Work out the finished part from the listing and answer in its coordinate system (mm). A direction names the side the tool comes from. Coordinates: 2 decimals unless noted, no trailing zeros. Order: outer loops, then holes, each group sorted by start corner. A loop starts at its lowest first (then second) coordinate and runs counter-clockwise, first axis right, second up. Notation, with made-up numbers: (-14.5, 79) -> (-2.5, 79) arc R19 cw to (-2.5, 90) -> close; hole circle Ø3 at (71.25, 16). An arc over 180 degrees is marked (long way). Write item = value, one per line. Start each with the question number.
Q1. The part is cut by section B-B, the plane z = -0.55. Determine the outline of the cut face in (x, y).
Q2. Straight lines are drawn through the part: L1, parallel to Y at x = 10.5, z = -0.85; L2, parallel to X at y = -12.75, z = -0.45; L3, parallel to Z at x = 11.25, y = 1. For each, find the intervals that lie inside material, in ascending order. Write a range as from..to.
Q3. Which of the six approach directions +Z, -Z, +X, -X, +Y, -Y give full straight-line access (tool end or side, diameter ignored) to faces 5 (the flat face through (9, -12, -0.9)), 6 (the flat face through (-0.1, 9.462, -0.5))?
Q4. The part is cut by section A-A, the plane y = 0.1. Determine the outline of the cut face in (x, z) (3 decimals).
Q5. The part is cut by section C-C, the plane y = -10.5. Determine the outline of the cut face in (x, z) (3 decimals).
Q6. Flat-ended cylindrical pins translate along their axes: pin 1 (2 mm diameter, centred on x = -10.5, y = -0.5, fed in from -Z); pin 2 (1.3 mm diameter, centred on x = -9.5, y = 0.5, fed in from +Z). Find the tip coordinate at first contact, or state that the pin passes through.
Q7. For a pull along Y with two mould halves and no side action, classify faces 1 (the flat face through (9, 0, -0.9)), 2 (the flat face through (0, -2, -0.975)), 3 (the flat face through (-9, -12, 0)), 4 (the cylindrical face through (11.9, -13.83, -0.46)) as +Y half, -Y half, draft (parallel to the pull), parting line (faces both ways), or undercut.
```python
from build123d import *

# Parameters (mm, degrees)
SKETCH3_W           = 25
SKETCH3_H           = 23.862
BOSS_EXTRUDE1_DEPTH = 0.9
FILLET1_R           = 2
SKETCH4_R           = 1.1
CUT_EXTRUDE1_DEPTH  = 20.089787846
BOSS_EXTRUDE2_DEPTH = 0.075
BOSS_EXTRUDE3_START = 0.075
BOSS_EXTRUDE3_DEPTH = 0.075


with BuildPart() as part:
    # Sketch3 → Boss-Extrude1 (new body)
    with BuildSketch(Plane.XY):
        with Locations((0, -2.469)):
            Rectangle(SKETCH3_W, SKETCH3_H)
    extrude(amount=-BOSS_EXTRUDE1_DEPTH)

    # Fillet1
    fillet1_edges = [part.edges().sort_by_distance(p)[0] for p in [
        (-12.5, 9.462, -0.45),
        (12.5, 9.462, -0.45),
        (12.5, -14.4, -0.45),
        (-12.5, -14.4, -0.45),
    ]]
    fillet(fillet1_edges, radius=FILLET1_R)

    # Sketch4 → Cut-Extrude1 (cut, through all)
    with BuildSketch(Plane.XY):
        with Locations((-10.5, 0.1)):
            Circle(SKETCH4_R)
        with Locations((-10.5, -12.4)):
            Circle(SKETCH4_R)
        with Locations((10.5, -12.4)):
            Circle(SKETCH4_R)
        with Locations((10.5, 0.1)):
            Circle(SKETCH4_R)
    extrude(amount=-CUT_EXTRUDE1_DEPTH, mode=Mode.SUBTRACT)

    # Sketch5 → Boss-Extrude2 (add)
    with BuildSketch(Plane.XY):
        with BuildLine():
            Line((12.5, 1.426649916), (12.5, 7.462))
            ThreePointArc((12.5, 7.462), (11.914213562, 8.876213562), (10.5, 9.462))
            Line((10.5, 9.462), (-10.5, 9.462))
            ThreePointArc((-10.5, 9.462), (-11.914213562, 8.876213562), (-12.5, 7.462))
            Line((-12.5, 7.462), (-12.5, 1.426649916))
            ThreePointArc((-12.5, 1.426649916), (-8.1, 0.1), (-12.5, -1.226649916))
            Line((-12.5, -1.226649916), (-12.5, -11.073350084))
            ThreePointArc((-12.5, -11.073350084), (-8.802943725, -10.702943725), (-9.173350084, -14.4))
            Line((-9.173350084, -14.4), (9.173350084, -14.4))
            ThreePointArc((9.173350084, -14.4), (8.802943725, -10.702943725), (12.5, -11.073350084))
            Line((12.5, -11.073350084), (12.5, -1.226649916))
            ThreePointArc((12.5, -1.226649916), (8.1, 0.1), (12.5, 1.426649916))
        make_face()
    extrude(amount=BOSS_EXTRUDE2_DEPTH)

    # Sketch6 → Boss-Extrude3 (add)
    with BuildSketch(Plane(origin=(0, 0, -0.9), x_dir=(-1, 0, 0), z_dir=(0, 0, -1)).offset(BOSS_EXTRUDE3_START)):
        with BuildLine():
            Line((12.5, 1.426649916), (12.5, 7.462))
            ThreePointArc((12.5, 7.462), (11.914213562, 8.876213562), (10.5, 9.462))
            Line((10.5, 9.462), (-10.5, 9.462))
            ThreePointArc((-10.5, 9.462), (-11.914213562, 8.876213562), (-12.5, 7.462))
            Line((-12.5, 7.462), (-12.5, 1.426649916))
            ThreePointArc((-12.5, 1.426649916), (-8.1, 0.1), (-12.5, -1.226649916))
            Line((-12.5, -1.226649916), (-12.5, -11.073350084))
            ThreePointArc((-12.5, -11.073350084), (-8.802943725, -10.702943725), (-9.173350084, -14.4))
            Line((-9.173350084, -14.4), (9.173350084, -14.4))
            ThreePointArc((9.173350084, -14.4), (8.802943725, -10.702943725), (12.5, -11.073350084))
            Line((12.5, -11.073350084), (12.5, -1.226649916))
            ThreePointArc((12.5, -1.226649916), (8.1, 0.1), (12.5, 1.426649916))
        make_face()
    extrude(amount=-BOSS_EXTRUDE3_DEPTH)


solid = part.part
```
Model answer:
q1.outline = (-12.5, -12.4) arc R2 ccw to (-10.5, -14.4) -> (10.5, -14.4) arc R2 ccw to (12.5, -12.4) -> (12.5, 7.46) arc R2 ccw to (10.5, 9.46) -> (-10.5, 9.46) arc R2 ccw to (-12.5, 7.46) -> close; hole circle Ø2.2 at (-10.5, -12.4); hole circle Ø2.2 at (-10.5, 0.1); hole circle Ø2.2 at (10.5, -12.4); hole circle Ø2.2 at (10.5, 0.1)
q2.L1 = -14.4..-13.5, -11.3..-1, 1.2..9.46
q2.L2 = -12.47..-11.54, -9.46..9.46, 11.54..12.47
q2.L3 = -0.9..0
q3.face_5 = -Z
q3.face_6 = +Z, -Z, +X, -X, +Y
q4.outline = (-12.5, -0.9) -> (-11.6, -0.9) -> (-11.6, 0) -> (-12.5, 0) -> close; (-9.4, -0.9) -> (-8.1, -0.9) -> (-8.1, -0.975) -> (8.1, -0.975) -> (8.1, -0.9) -> (9.4, -0.9) -> (9.4, 0) -> (8.1, 0) -> (8.1, 0.075) -> (-8.1, 0.075) -> (-8.1, 0) -> (-9.4, 0) -> close; (11.6, -0.9) -> (12.5, -0.9) -> (12.5, 0) -> (11.6, 0) -> close
q5.outline = (-12.5, -0.975) -> (-11.966, -0.975) -> (-11.966, -0.9) -> (-9.034, -0.9) -> (-9.034, -0.975) -> (9.034, -0.975) -> (9.034, -0.9) -> (11.966, -0.9) -> (11.966, -0.975) -> (12.5, -0.975) -> (12.5, 0.075) -> (11.966, 0.075) -> (11.966, 0) -> (9.034, 0) -> (9.034, 0.075) -> (-9.034, 0.075) -> (-9.034, 0) -> (-11.966, 0) -> (-11.966, 0.075) -> (-12.5, 0.075) -> close
q6.pin_1 = -0.9
q6.pin_2 = 0
q7.face_1 = undercut
q7.face_2 = draft
q7.face_3 = undercut
q7.face_4 = -Y half
